Here's how the part is built. I have some questions about the finished solid (model axes, mm). Face numbers are marked on the shaded views. A direction names the side the tool comes from. Coordinates: 2 decimals unless noted, no trailing zeros. Loops run counter-clockwise (first coordinate to the right, second up) from the corner with the lowest first, then second, coordinate; pieces in that order, holes last. Notation, with made-up numbers: (-7.5, 71.25) -> (33.5, 71.25) arc R29 cw to (33.5, 105.25) -> close; hole circle Ø10 at (37.25, 62). An arc over 180 degrees is marked (long way). Answer as a JSON object with one key per item and string values. Group by question number.
Q1. I want a section at D-D on z = 7.5. Write out the boundary of the cut face in (x, y), then the cut area to 3 significant figures.
Q2. I need wall thicknesses on line 1 (X direction, y = -8, z = 7); line 2 (X direction, y = -0.5, z = 0); line 3 (Y direction, x = 3, z = 0). Which ranges of each line are inside material? Lowest first, please.
Q3. I want a section at B-B on y = 7. Write out the boundary of the cut face in (x, z).
Q4. I'm going to push flat-ended pins straight in: pin 1 (8 mm diameter, centred on x = 18.5, y = -14.5, fed in from +Z); pin 2 (6 mm diameter, centred on y = -6.5, z = -13.5, fed in from +X); pin 3 (8 mm diameter, centred on x = 18, y = -6, fed in from -Z). Where does each tip first touch, or does it pass through?
Q5. On a 3-axis mill with a long thin cutter (end or side, diameter ignored), from which of +Z, -Z, +X, -X, +Y, -Y can I reach the whole of each face in a straight line? I mean the marked faces 1, 2 and 3. Say none if no direction works.
Q6. I want a section at A-A on z = 0. Write out the boundary of the cut face in (x, y), then the cut area to 3 significant figures.
Q7. I want a section at C-C on x = 43. Write out the boundary of the cut face in (y, z), then the cut area to 3 significant figures.
```python
from build123d import *

# Parameters (mm, degrees)
SKETCH_1_R               = 16.5
EXTRUDE_1_DEPTH          = 22.7
SKETCH_2_R               = 18.5
EXTRUDE_2_DEPTH          = 24
SKETCH_3_R               = 6.5
EXTRUDE_3_DEPTH          = 8.5
SKETCH_5_R               = 1.5
CUT_EXTRUDE_2_DEPTH      = 10
SKETCH_2_2_R             = 18.5
EXTRUDE_4_DEPTH          = 26.5
SKETCH_3_2_R             = 6.5
EXTRUDE_5_DEPTH          = 6
SKETCH_9_R               = 3
EXTRUDE_6_DEPTH          = 15.5
CUT_EXTRUDE_3_DEPTH      = 76.385608706
CUT_EXTRUDE_3_DEPTH_BACK = 12
SKETCH_11_R              = 6
EXTRUDE_7_DEPTH          = 2
FILLET_1_R               = 0.5


with BuildPart() as part:
    # 草图1 → 凸台-拉伸1 (new body)
    with BuildSketch(Plane(origin=(0, 0, 0), x_dir=(0, 0, -1), z_dir=(1, 0, 0))):
        Circle(SKETCH_1_R)
    extrude(amount=EXTRUDE_1_DEPTH)

    # 草图2 → 凸台-拉伸2 (add)
    with BuildSketch(Plane(origin=(22.7, 0, 0), x_dir=(0, 0, -1), z_dir=(1, 0, 0))):
        Circle(SKETCH_2_R)
    extrude(amount=EXTRUDE_2_DEPTH)

    # 草图3 → 凸台-拉伸3 (add)
    with BuildSketch(Plane(origin=(46.7, 0, 0), x_dir=(0, 0, -1), z_dir=(1, 0, 0))):
        with Locations((0, 7)):
            Circle(SKETCH_3_R)
    extrude(amount=EXTRUDE_3_DEPTH)

    # 草图5 → 切除-拉伸2 (cut)
    with BuildSketch(Plane(origin=(46.7, 0, 0), x_dir=(0, 0, -1), z_dir=(1, 0, 0))):
        with Locations((-15.5, 0)):
            Circle(SKETCH_5_R)
        with Locations((-7.75, 13.423393759)):
            Circle(SKETCH_5_R)
        with Locations((7.75, 13.423393759)):
            Circle(SKETCH_5_R)
        with Locations((15.5, 0)):
            Circle(SKETCH_5_R)
        with Locations((7.75, -13.423393759)):
            Circle(SKETCH_5_R)
        with Locations((-7.75, -13.423393759)):
            Circle(SKETCH_5_R)
    extrude(amount=-CUT_EXTRUDE_2_DEPTH, mode=Mode.SUBTRACT)

    # 草图2<2> → 凸台-拉伸4 (add)
    with BuildSketch(Plane(origin=(22.7, 0, 0), x_dir=(0, 0, -1), z_dir=(1, 0, 0))):
        Circle(SKETCH_2_2_R)
    extrude(amount=EXTRUDE_4_DEPTH)

    # 草图3<2> → 凸台-拉伸5 (add)
    with BuildSketch(Plane(origin=(46.7, 0, 0), x_dir=(0, 0, -1), z_dir=(1, 0, 0))):
        with Locations((0, 7)):
            Circle(SKETCH_3_2_R)
    extrude(amount=EXTRUDE_5_DEPTH)

    # 草图9 → 凸台-拉伸6 (add)
    with BuildSketch(Plane(origin=(55.2, 0, 0), x_dir=(0, 0, -1), z_dir=(1, 0, 0))):
        with Locations((0, 7)):
            Circle(SKETCH_9_R)
    extrude(amount=EXTRUDE_6_DEPTH)

    # 草图10 → 切除-拉伸3 (cut, two sides: drawn at the far end of the back side and taken through both)
    with BuildSketch(Plane(origin=(70.7, 0, 0), x_dir=(0, 0, -1), z_dir=(1, 0, 0)).offset(-CUT_EXTRUDE_3_DEPTH_BACK)):
        Polygon((-80.474239871, 9.6), (-1.496662955, 9.6), (1.496662955, 9.6), (80.474239871, 9.6), (80.474239871, 167.555153833), (-80.474239871, 167.555153833), align=None)
    extrude(amount=CUT_EXTRUDE_3_DEPTH + CUT_EXTRUDE_3_DEPTH_BACK, mode=Mode.SUBTRACT)

    # 草图11 → 凸台-拉伸7 (add)
    with BuildSketch(Plane.ZY):
        Circle(SKETCH_11_R)
    extrude(amount=EXTRUDE_7_DEPTH)

    # 圆角1
    fillet_1_edges = [part.edges().sort_by_distance(p)[0] for p in [
        (-2, 0, -6),
    ]]
    fillet(fillet_1_edges, radius=FILLET_1_R)


solid = part.part
```
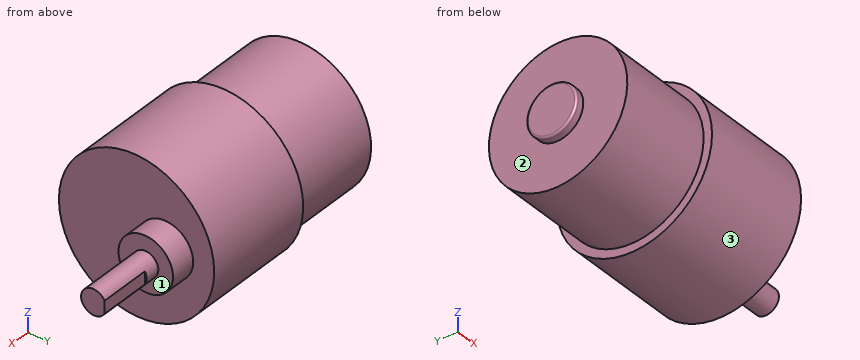
Result set:
{
 "1": {"outline": "(0, -14.7) -> (22.7, -14.7) -> (22.7, -16.91) -> (49.2, -16.91) -> (49.2, 16.91) -> (22.7, 16.91) -> (22.7, 14.7) -> (0, 14.7) -> close", "area": "1,560 mm²"},
 "2": {"line 1": "x = 0 to 49.2", "line 2": "x = -2 to 49.2", "line 3": "y = -16.5 to 16.5"},
 "3": {"outline": "(0, -14.94) -> (22.7, -14.94) -> (22.7, -17.12) -> (49.2, -17.12) -> (49.2, -6.5) -> (55.2, -6.5) -> (55.2, -3) -> (70.7, -3) -> (70.7, 3) -> (55.2, 3) -> (55.2, 6.5) -> (49.2, 6.5) -> (49.2, 17.12) -> (22.7, 17.12) -> (22.7, 14.94) -> (0, 14.94) -> close"},
 "4": {"pin 1": "stops at z = 12.73", "pin 2": "stops at x = 49.2", "pin 3": "stops at z = -16.38"},
 "5": {"face 1": "+X", "face 2": "-X", "face 3": "+X, -X"},
 "6": {"outline": "(-2, -5.5) arc R0.5 ccw to (-1.5, -6) -> (0, -6) -> (0, -16.5) -> (22.7, -16.5) -> (22.7, -18.5) -> (49.2, -18.5) -> (49.2, 0.5) -> (55.2, 0.5) -> (55.2, 4) -> (70.7, 4) -> (70.7, 9.6) -> (58.7, 9.6) -> (58.7, 10) -> (55.2, 10) -> (55.2, 13.5) -> (49.2, 13.5) -> (49.2, 18.5) -> (22.7, 18.5) -> (22.7, 16.5) -> (0, 16.5) -> (0, 6) -> (-1.5, 6) arc R0.5 ccw to (-2, 5.5) -> close", "area": "1,920 mm²"},
 "7": {"outline": "circle Ø37 at (0, 0)", "area": "1,080 mm²"}
}
